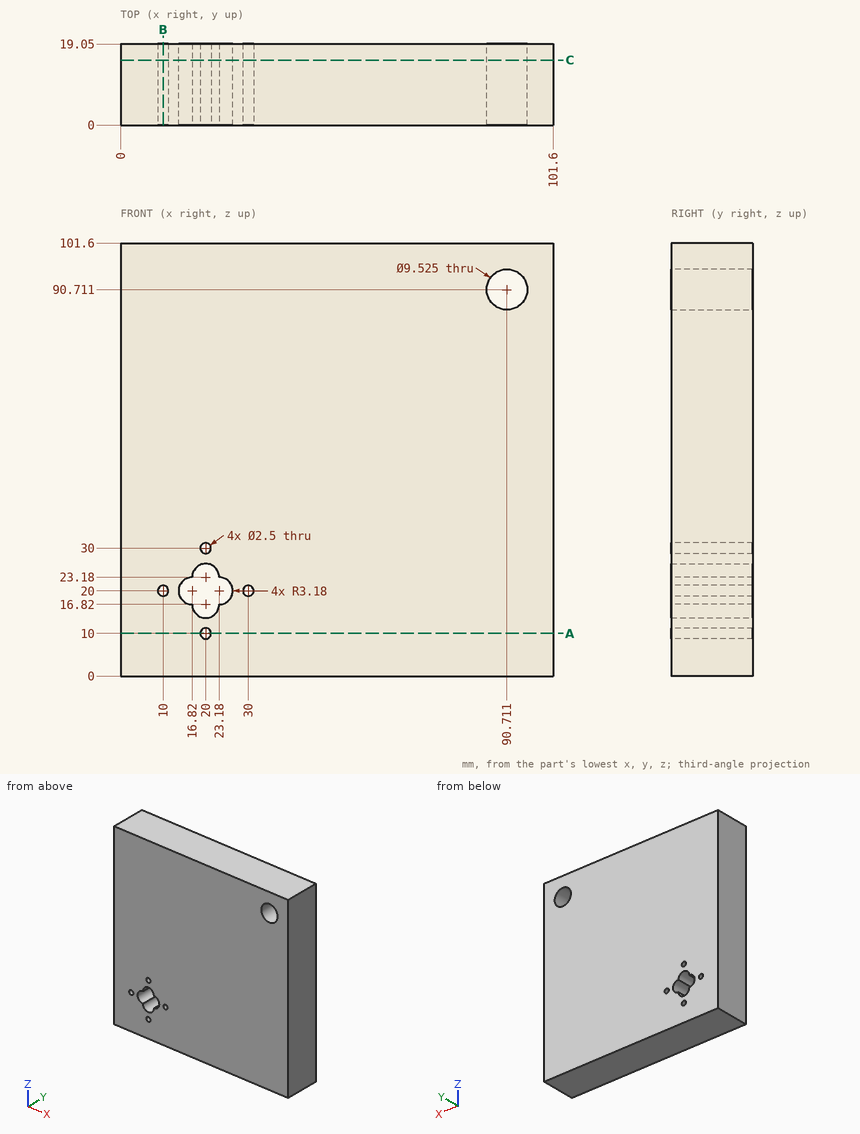
For this review, use the dimensioned drawing (mm, ordinates from the lowest corner) and the shaded views. Round coordinates to 2 decimals unless told otherwise and drop trailing zeros. Order: outer loops, then holes, each group sorted by start corner. A loop starts at its lowest first (then second) coordinate and runs counter-clockwise, first axis right, second up.
1) Consider section C-C (y = 15.25). Count the separate pieces of the cut face and the enclosed holes in it, plus the area to 3 significant figures.
The answers:
separate pieces: 1
enclosed holes: 6
area: 10,100 mm2
2) Clearance check with flat-ended pins moving along their axes: pin 1 Ø4 at (x, z) = (10, 20) entering from -Y; pin 2 Ø5.5 at (x, z) = (90.71, 90.71) entering from +Y (3 decimals). State where each tip first meets the part, or that it passes through.
The answers:
pin 1: stops at y = 0
pin 2: passes through
3) Consider section B-B (x = 10). State the section outline as (y, z) points, plus the area to 3 significant figures.
The answers:
outline: (0, 0) - (19.05, 0) - (19.05, 18.75) - (0, 18.75) - close; (0, 21.25) - (19.05, 21.25) - (19.05, 101.6) - (0, 101.6) - close
area: 1,890 mm2
4) Consider section A-A (z = 10). State the section outline as (x, y) points, plus the area to 3 significant figures.
The answers:
outline: (0, 0) - (18.75, 0) - (18.75, 19.05) - (0, 19.05) - close; (21.25, 0) - (101.6, 0) - (101.6, 19.05) - (21.25, 19.05) - close
area: 1,890 mm2
5) For L1, parallel to X at y = 9.5, z = 20; L2, parallel to X at y = 15.75, z = 30, list the stretches that pass through material, from the lowest coordinate up.
The answers:
L1: x = 0 to 8.75, 11.25 to 13.64, 26.36 to 28.75, 31.25 to 101.6
L2: x = 0 to 18.75, 21.25 to 101.6
